Design review of the part built by this model. Coordinates are the model's own, in mm. Face numbers are marked on the shaded views. A direction names the side the tool comes from. Coordinates: 2 decimals unless noted, no trailing zeros. Loops run counter-clockwise (first coordinate to the right, second up) from the corner with the lowest first, then second, coordinate; pieces in that order, holes last.
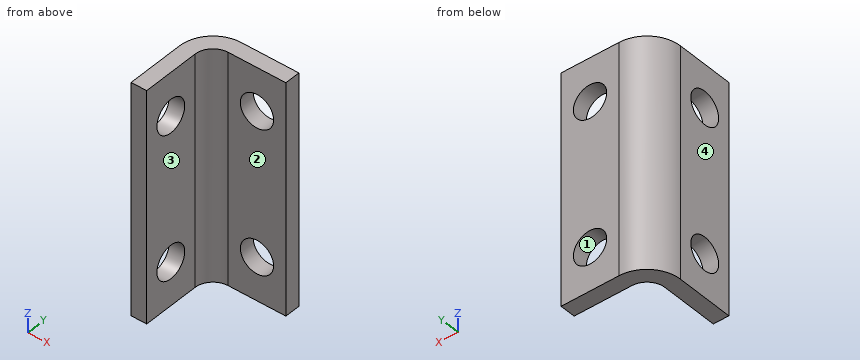
from build123d import *

# Parameters (mm, degrees)
F1_DEPTH = 25.4
F2_R     = 1.8288
F3_DEPTH = 1.70942
F4_R     = 1.8288
F5_DEPTH = 1.70942
F6_R     = 1.98374
F7_R     = 3.69316


with BuildPart() as f1:
    # F0 (on Top) → F1 (new body)
    with BuildSketch(Plane.XY):
        Polygon((-1.70942, -8.33374), (0, -8.33374), (0, 0), (8.33374, 0), (8.33374, 1.70942), (-1.70942, 1.70942), align=None)
    extrude(amount=F1_DEPTH)

    # F2 (on face) → F3 (cut, through all)
    with BuildSketch(Plane.XZ):
        with Locations((5.15874, 20.6375)):
            Circle(F2_R)
        with Locations((5.15874, 4.7625)):
            Circle(F2_R)
    extrude(amount=-F3_DEPTH, mode=Mode.SUBTRACT)

    # F4 (on face) → F5 (cut, through all)
    with BuildSketch(Plane.YZ):
        with Locations((-5.15874, 20.6375)):
            Circle(F4_R)
        with Locations((-5.15874, 4.7625)):
            Circle(F4_R)
    extrude(amount=-F5_DEPTH, mode=Mode.SUBTRACT)

    # F6
    f6_edges = [f1.edges().sort_by_distance(p)[0] for p in [
        (0, 0, 12.7),
    ]]
    fillet(f6_edges, radius=F6_R)

    # F7
    f7_edges = [f1.edges().sort_by_distance(p)[0] for p in [
        (-1.70942, 1.70942, 12.7),
    ]]
    fillet(f7_edges, radius=F7_R)


solid = f1.part
Q1. Take a section at C-C, the plane z = 11.5. Write out the cut boundary in (x, y).
Q2. For line 1 (Y direction, x = 3, z = 14.5); line 2 (X direction, y = -6.5, z = 24.25); line 3 (Z direction, x = -0.25, y = -5.75), list the stretches that pass through material, from the lowest coordinate up.
Q3. The part is to be moulded in two halves that separate along Z. For the marked faces 1 and 2, say which applies: pulls with the +Z half, pulls with the -Z half, needs draft (parallel to the pull), parting line crosses it, or undercut.
Q4. Take a section at A-A, the plane x = 4.75. Write out the cut boundary in (y, z).
Q5. Take a section at B-B, the plane y = -3.75. Write out the cut boundary in (x, z).
Q6. Machinability: for the marked faces 3 and 4, which of the approach directions +Z, -Z, +X, -X, +Y, -Y give a long, thin tool a straight path to every point of the face, cutting with its end or side? Answer none if there is none.
Q7. Take a section at D-D, the plane z = 4.5. Write out the cut boundary in (x, y), then the cut area to 3 significant figures.
Q8. Clearance check with flat-ended pins moving along their axes: pin 1 Ø2 at (x, z) = (5.16, 4.76) entering from +Y; pin 2 Ø1.5 at (x, z) = (1.5, 5) entering from -Y; pin 3 Ø5 at (y, z) = (-5.5, 11.5) entering from +X; pin 4 Ø1.5 at (y, z) = (-1, 7.5) entering from +X. State where each tip first meets the part, or that it passes through.
Entries:
1. outline: (-1.71, -8.33) - (0, -8.33) - (0, -1.98) arc R1.98 cw to (1.98, 0) - (8.33, 0) - (8.33, 1.71) - (1.98, 1.71) arc R3.69 ccw to (-1.71, -1.98) - close
2. line 1: y = 0 to 1.71
2. line 2: x = -1.71 to 0
2. line 3: z = 0 to 3.03, 6.49 to 18.91, 22.37 to 25.4
3. face 1: undercut
3. face 2: needs draft
4. outline: (0, 0) - (1.71, 0) - (1.71, 2.98) - (0, 2.98) - close; (0, 6.55) - (1.71, 6.55) - (1.71, 18.85) - (0, 18.85) - close; (0, 22.42) - (1.71, 22.42) - (1.71, 25.4) - (0, 25.4) - close
5. outline: (-1.71, 0) - (0, 0) - (0, 3.6) - (-1.71, 3.6) - close; (-1.71, 5.93) - (0, 5.93) - (0, 19.47) - (-1.71, 19.47) - close; (-1.71, 21.8) - (0, 21.8) - (0, 25.4) - (-1.71, 25.4) - close
6. face 3: +Z, -Z, +X, -Y
6. face 4: +Z, -Z, -X, +Y, -Y
7. outline: (-1.71, -8.33) - (0, -8.33) - (0, -6.97) - (-1.71, -6.97) - close; (-1.71, -3.35) - (0, -3.35) - (0, -1.98) arc R1.98 cw to (1.98, 0) - (3.35, 0) - (3.35, 1.71) - (1.98, 1.71) arc R3.69 ccw to (-1.71, -1.98) - close; (6.97, 0) - (8.33, 0) - (8.33, 1.71) - (6.97, 1.71) - close
7. area: 17.0 mm2
8. pin 1: passes through
8. pin 2: stops at y = -0.43
8. pin 3: stops at x = 0
8. pin 4: stops at x = 1.02
